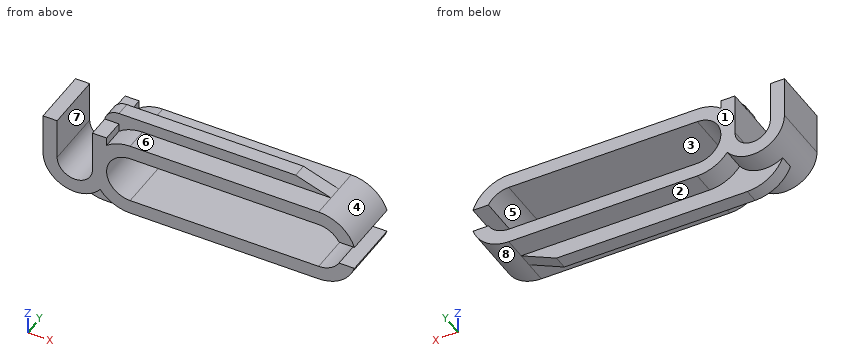
```python
from build123d import *

# Parameters (mm, degrees)
BOSS_EXTRUDE1_DEPTH = 5
CUT_EXTRUDE1_DEPTH  = 6
SKETCH4_W           = 4
SKETCH4_H           = 2
CUT_EXTRUDE2_DEPTH  = 6
BOSS_EXTRUDE2_DEPTH = 5
CUT_EXTRUDE3_DEPTH  = 6
BOSS_EXTRUDE3_DEPTH = 0.6
BOSS_EXTRUDE4_DEPTH = 0.6


with BuildPart() as part:
    # Sketch1 → Boss-Extrude1 (new body)
    with BuildSketch(Plane(origin=(0, 0, 0), x_dir=(1, 0, 0), z_dir=(0, 1, 0))):
        with BuildLine():
            Line((-8, 3.2), (8, 3.2))
            ThreePointArc((8, 3.2), (11.2, 0), (8, -3.2))
            Line((8, -3.2), (-8, -3.2))
            ThreePointArc((-8, -3.2), (-11.2, 0), (-8, 3.2))
        make_face()
    extrude(amount=BOSS_EXTRUDE1_DEPTH)

    # Sketch3 → Cut-Extrude1 (cut, through all)
    with BuildSketch(Plane(origin=(0, 5, 0), x_dir=(1, 0, 0), z_dir=(0, 1, 0))):
        with BuildLine():
            Line((-8, 2), (8, 2))
            ThreePointArc((8, 2), (10, 0), (8, -2))
            Line((8, -2), (-8, -2))
            ThreePointArc((-8, -2), (-10, 0), (-8, 2))
        make_face()
    extrude(amount=-CUT_EXTRUDE1_DEPTH, mode=Mode.SUBTRACT)

    # Sketch4 → Cut-Extrude2 (cut, through all)
    with BuildSketch(Plane(origin=(0, 5, 0), x_dir=(1, 0, 0), z_dir=(0, 1, 0))):
        with Locations((10.5, 0)):
            Rectangle(SKETCH4_W, SKETCH4_H)
    extrude(amount=-CUT_EXTRUDE2_DEPTH, mode=Mode.SUBTRACT)

    # Sketch5 → Boss-Extrude2 (add)
    with BuildSketch(Plane.XZ):
        with BuildLine():
            Line((-10, -0.3), (-10, 3.2))
            Line((-10, 3.2), (-15.4, 3.2))
            Line((-15.4, 3.2), (-15.4, -0.3))
            ThreePointArc((-15.4, -0.3), (-12.7, -3), (-10, -0.3))
        make_face()
    extrude(amount=-BOSS_EXTRUDE2_DEPTH)

    # Sketch7 → Cut-Extrude3 (cut, through all)
    with BuildSketch(Plane.XZ):
        with BuildLine():
            Line((-14.2, -0.3), (-14.2, 3.2))
            Line((-14.2, 3.2), (-11.2, 3.2))
            Line((-11.2, 3.2), (-11.2, -0.3))
            ThreePointArc((-11.2, -0.3), (-12.7, -1.8), (-14.2, -0.3))
        make_face()
    extrude(amount=-CUT_EXTRUDE3_DEPTH, mode=Mode.SUBTRACT)

    # Sketch8 → Boss-Extrude3 (add, symmetric)
    with BuildSketch(Plane(origin=(0, 2.5, 0), x_dir=(1, 0, 0), z_dir=(0, 1, 0))):
        with BuildLine():
            Line((-11.2, 4.6), (5, 4.6))
            Line((5, 4.6), (8, 3.2))
            Line((8, 3.2), (-8, 3.2))
            ThreePointArc((-8, 3.2), (-9.423654515, 2.86586947), (-10.550005007, 1.933254888))
            ThreePointArc((-10.550005007, 1.933254888), (-12.253704481, 2.962859424), (-14.2, 2.544994432))
            ThreePointArc((-14.2, 2.544994432), (-13.018175451, 4.036985667), (-11.2, 4.6))
        make_face()
    extrude(amount=BOSS_EXTRUDE3_DEPTH, both=True)

    # Sketch9 → Boss-Extrude4 (add, symmetric)
    with BuildSketch(Plane(origin=(0, 2.5, 0), x_dir=(1, 0, 0), z_dir=(0, 1, 0))):
        with BuildLine():
            Line((-8, -3.2), (8, -3.2))
            Line((8, -3.2), (5, -4.2))
            Line((5, -4.2), (-10, -4.2))
            ThreePointArc((-10, -4.2), (-10.781024968, -3.917229961), (-11.2, -3.2))
            Line((-11.2, -3.2), (-10, -3.2))
            Line((-10, -3.2), (-10, -2.497999199))
            ThreePointArc((-10, -2.497999199), (-9.059811908, -3.019403703), (-8, -3.2))
        make_face()
    extrude(amount=BOSS_EXTRUDE4_DEPTH, both=True)


solid = part.part
```
Check sheet for the modelled part. Datum: model origin and axes. Units: mm. Face numbers are marked on the shaded views. A direction names the side the tool comes from. Coordinates: 2 decimals unless noted, no trailing zeros. Write each loop counter-clockwise with the first axis right and the second up, starting at its lowest first coordinate (ties: lowest second). Pieces come first, ordered by that corner, then holes. Notation, with made-up numbers: (5, 79) -> (63, 79) arc R21 cw to (63, 94) -> close; hole circle Ø2 at (30.25, 35.5). An arc over 180 degrees is marked (long way). Use a Markdown table: item, result.
1. Sectioned sample at A-A (x = -1). Enter the section's corners in (y, z), plus the area to 3 significant figures.
Reported:
| item | result |
|---|---|
| outline | (0, -3.2) -> (1.9, -3.2) -> (1.9, -4.6) -> (3.1, -4.6) -> (3.1, -3.2) -> (5, -3.2) -> (5, -2) -> (0, -2) -> close; (0, 2) -> (5, 2) -> (5, 3.2) -> (3.1, 3.2) -> (3.1, 4.2) -> (1.9, 4.2) -> (1.9, 3.2) -> (0, 3.2) -> close |
| area | 14.9 mm2 |
2. Release check for a two-part mould opening along Z. For the marked faces 1, 2 and 3 record: pulls with the +Z half, pulls with the -Z half, needs draft (parallel to the pull), parting line crosses it, or undercut.
Reported:
| item | result |
|---|---|
| face 1 | needs draft |
| face 2 | pulls with the -Z half |
| face 3 | undercut |
3. Sectioned sample at C-C (y = 1.6). Enter the section's corners in (x, z), plus the area to 3 significant figures.
Reported:
| item | result |
|---|---|
| outline | (-15.4, -0.3) arc R2.7 ccw to (-10.55, -1.93) arc R3.2 ccw to (-8, -3.2) -> (8, -3.2) arc R3.2 ccw to (11.04, -1) -> (9.73, -1) arc R2 cw to (8, -2) -> (-8, -2) arc R2 cw to (-8, 2) -> (8, 2) arc R2 cw to (9.73, 1) -> (11.04, 1) arc R3.2 ccw to (8, 3.2) -> (-8, 3.2) arc R3.2 ccw to (-10, 2.5) -> (-10, 3.2) -> (-11.2, 3.2) -> (-11.2, -0.3) arc R1.5 cw to (-14.2, -0.3) -> (-14.2, 3.2) -> (-15.4, 3.2) -> close |
| area | 68.1 mm2 |
4. Go/stop test with flat-tipped pins: pin 1 Ø1 at (x, y) = (-3.5, 1) entering from +Z; pin 2 Ø3 at (y, z) = (4.5, -3.5) entering from -X; pin 3 Ø0.6 at (y, z) = (1, 3) entering from +X. Record where each tip stops, or that it passes through.
Reported:
| item | result |
|---|---|
| pin 1 | stops at z = 3.2 |
| pin 2 | stops at x = -14.8 |
| pin 3 | stops at x = 9.72 |
5. Tool access check on the marked faces 4, 5, 6, 7 and 8. Record the directions out of +Z, -Z, +X, -X, +Y, -Y that give a thin tool (end or side, any length) a straight path to the whole face; none if there is none.
Reported:
| item | result |
|---|---|
| face 4 | +Z, +X, +Y, -Y |
| face 5 | +Y, -Y |
| face 6 | +Z, +X, -X, -Y |
| face 7 | +Z, +Y, -Y |
| face 8 | -Z, +X, +Y, -Y |
6. Sectioned sample at B-B (z = 0). Enter the section's corners in (x, y).
Reported:
| item | result |
|---|---|
| outline | (-15.4, 0) -> (-14.2, 0) -> (-14.2, 5) -> (-15.4, 5) -> close; (-11.2, 0) -> (-10, 0) -> (-10, 5) -> (-11.2, 5) -> close |
7. Scan lines: line 1 along Z through (x, y) = (3.75, 2.4); line 2 along Z through (x, y) = (-2.25, 1.45); line 3 along X through (y, z) = (4.7, 0). Record each from-to range of solid material in increasing order.
Reported:
| item | result |
|---|---|
| line 1 | z = -4.6 to -2, 2 to 4.2 |
| line 2 | z = -3.2 to -2, 2 to 3.2 |
| line 3 | x = -15.4 to -14.2, -11.2 to -10 |
8. Sectioned sample at D-D (x = -11.75). Enter the section's corners in (y, z), plus the area to 3 significant figures.
Reported:
| item | result |
|---|---|
| outline | (0, -2.83) -> (1.9, -2.83) -> (1.9, -4.55) -> (3.1, -4.55) -> (3.1, -2.83) -> (5, -2.83) -> (5, -1.46) -> (0, -1.46) -> close |
| area | 8.90 mm2 |
